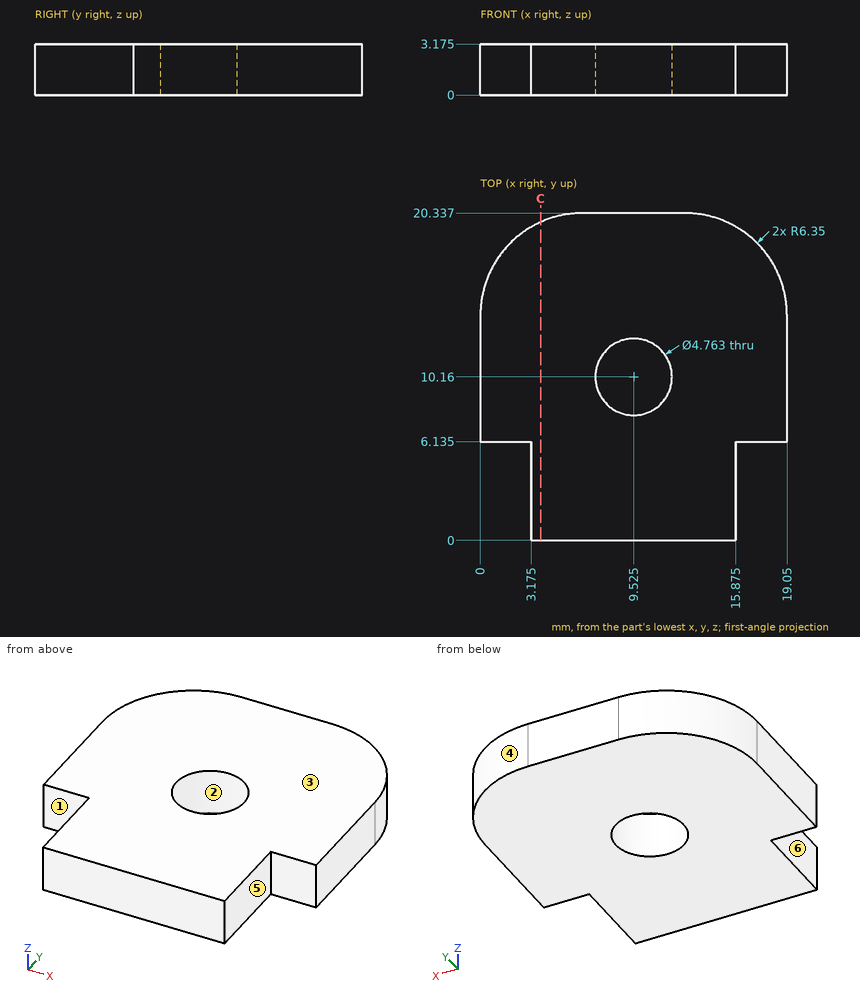
Design review of the part shown in the three views and the two pictorial views. Dimensions are in mm from the part's minimum x, y and z. A direction names the side the tool comes from. Give positions to 0.01 mm unless a question says otherwise; leave off trailing zeros. Loops run counter-clockwise (first coordinate to the right, second up) from the corner with the lowest first, then second, coordinate; pieces in that order, holes last. Notation, with made-up numbers: M 75.5,6.5 L 107.5,6.5 A20 cw 107.5,16.5 Z; hole C -24.75,-9.75 d4. An arc over 180 degrees is marked long. Put each result on its own line as item: value. Start each with the question number.
(1) For pin 1 (1.6 mm diameter, centred on y = 3, z = 2, fed in from -X) (1 decimal), flat-tipped, find the tip position at first contact; note if it passes through.
(2) Add section C-C, the plane x = 3.75. Write out the cut boundary in (y, z) (1 decimal).
(3) Machinability: for the marked faces 4, 5 and 6, which of the approach directions +Z, -Z, +X, -X, +Y, -Y give a long, thin tool a straight path to every point of the face, cutting with its end or side? Answer none if there is none.
(4) The part is to be moulded in two halves that separate along Y. For the marked faces 1, 2 and 3, say which applies: +Y half, -Y half, draft (parallel to the pull), parting line (faces both ways), or undercut.
(5) Wall thickness on L1, parallel to X at y = 1.5, z = 0.6 (1 decimal); L2, parallel to X at y = 17.25, z = 1.1; L3, parallel to Y at x = 3, z = 2.7 (1 decimal): over which ranges is each line inside the solid? List them lowest first.
Result:
1. pin 1: stops at x = 3.2
2. outline: M 0,0 L 19.8,0 L 19.8,3.2 L 0,3.2 Z
3. face 4: +Z, -Z, +X, +Y
3. face 5: +Z, -Z, +X, -Y
3. face 6: +Z, -Z, -X, -Y
4. face 1: -Y half
4. face 2: undercut
4. face 3: draft
5. L1: x = 3.2 to 15.9
5. L2: x = 0.9 to 18.15
5. L3: y = 6.1 to 19.4
